Check sheet for the modelled part. Datum: model origin and axes. Units: mm. Round coordinates to 2 decimals unless told otherwise and drop trailing zeros. Write each loop counter-clockwise with the first axis right and the second up, starting at its lowest first coordinate (ties: lowest second). Pieces come first, ordered by that corner, then holes.
Item 1: Material ranges on line 1 along X through (y, z) = (52.5, 1.5); line 2 along Y through (x, z) = (-206, 2.25); line 3 along Y through (x, z) = (-303, 4.5), recorded low to high.
Item 2: Section check B-B, the plane x = -58.5. Record the cut outline in (y, z).
Item 3: Section check A-A, the plane y = 93.5. Record the cut outline in (x, z).
Item 4: Section check D-D, the plane x = 269. Record the cut outline in (y, z), plus the area to 3 significant figures.
Item 5: Depth check by flat-ended pin: pin 1 (1 mm diameter, centred on x = 224.5, z = 1, fed in from +Y); pin 2 (3.5 mm diameter, centred on x = 45, z = 0.5, fed in from +Y); pin 3 (3 mm diameter, centred on y = 11, z = -1.5, fed in from -X); pin 4 (4 mm diameter, centred on x = 169.5, y = 18.5, fed in from -Z). Enter the tip coordinate at first touch or a pass-through.
Item 6: Release check for a two-part mould opening along Y. For faces 1 (the flat face through (234.723, 149.645, 0.067)), 2 (the flat face through (80, 89, 4.762)), 3 (the cylindrical face through (-214.43, 9.3, -0.07)) record: pulls with the +Y half, pulls with the -Y half, needs draft (parallel to the pull), parting line crosses it, or undercut.
Item 7: Section check C-C, the plane z = 0. State how many separate pieces and enclosed holes the cut face has, plus the area to 3 significant figures.
from build123d import *

# Parameters (mm, degrees)
SKETCH2_R           = 7.239
BOSS_EXTRUDE1_DEPTH = 4.7625
FILLET1_R           = 25.4
FILLET2_R           = 101.6
SKETCH3_W           = 25.4
SKETCH3_H           = 27.686
CUT_EXTRUDE1_DEPTH  = 10.525
SKETCH5_W           = 88.9
SKETCH5_H           = 114.3
CUT_EXTRUDE2_DEPTH  = 10.525
CUT_EXTRUDE3_DEPTH  = 10.525


with BuildPart() as part:
    # Sketch2 → Boss-Extrude1 (new body, symmetric)
    with BuildSketch(Plane.XY):
        Polygon((-340, 26.400000032), (-340, 121.400000032), (-75, 165), (135, 176.400000032), (340, 121.400000032), (340, 26.400000032), (340, 0), (-340, 0), align=None)
        with Locations((-208.682, 13.700000032)):
            Circle(SKETCH2_R, mode=Mode.SUBTRACT)
        with Locations((-77.364, 13.700000032)):
            Circle(SKETCH2_R, mode=Mode.SUBTRACT)
        with Locations((53.954, 13.700000032)):
            Circle(SKETCH2_R, mode=Mode.SUBTRACT)
        with Locations((185.126699107, 12.7)):
            Circle(SKETCH2_R, mode=Mode.SUBTRACT)
        with Locations((306.284699107, 10.414)):
            Circle(SKETCH2_R, mode=Mode.SUBTRACT)
        with Locations((168.225103232, 12.7)):
            Circle(SKETCH2_R, mode=Mode.SUBTRACT)
    extrude(amount=BOSS_EXTRUDE1_DEPTH, both=True)

    # Fillet1
    fillet1_edges = [part.edges().sort_by_distance(p)[0] for p in [
        (-340, 121.400000032, 0),
        (340, 121.400000032, 0),
    ]]
    fillet(fillet1_edges, radius=FILLET1_R)

    # Fillet2
    fillet2_edges = [part.edges().sort_by_distance(p)[0] for p in [
        (-75, 165, 0),
        (135, 176.400000032, 0),
    ]]
    fillet(fillet2_edges, radius=FILLET2_R)

    # Sketch3 → Cut-Extrude1 (cut, through all)
    with BuildSketch(Plane.XY.offset(4.7625)):
        with Locations((-327.3, 13.843)):
            Rectangle(SKETCH3_W, SKETCH3_H)
    extrude(amount=-CUT_EXTRUDE1_DEPTH, mode=Mode.SUBTRACT)

    # Sketch5 → Cut-Extrude2 (cut, through all)
    with BuildSketch(Plane.XY.offset(4.7625)):
        with Locations((-36.66848567, 86.296499999)):
            Rectangle(SKETCH5_W, SKETCH5_H)
    extrude(amount=-CUT_EXTRUDE2_DEPTH, mode=Mode.SUBTRACT)

    # Sketch8 → Cut-Extrude3 (cut, through all)
    with BuildSketch(Plane.XY.offset(4.7625)):
        with BuildLine():
            Line((161, 37.4), (162, 37.4))
            ThreePointArc((162, 37.4), (164.1, 35.3), (162, 33.2))
            Line((162, 33.2), (161, 33.2))
            ThreePointArc((161, 33.2), (158.9, 35.3), (161, 37.4))
        make_face()
        with BuildLine():
            Line((47, 33.2), (44, 33.2))
            ThreePointArc((44, 33.2), (41.9, 35.3), (44, 37.4))
            Line((44, 37.4), (47, 37.4))
            ThreePointArc((47, 37.4), (49.1, 35.3), (47, 33.2))
        make_face()
    extrude(amount=-CUT_EXTRUDE3_DEPTH, mode=Mode.SUBTRACT)


solid = part.part
Values found:
1. line 1: x = -340 to -81.12, 7.78 to 340
1. line 2: y = 0 to 6.98, 20.42 to 143.45
1. line 3: y = 0 to 127.49
2. outline: (0, -4.76) - (29.15, -4.76) - (29.15, 4.76) - (0, 4.76) - close; (143.45, -4.76) - (165.9, -4.76) - (165.9, 4.76) - (143.45, 4.76) - close
3. outline: (-340, -4.76) - (-81.12, -4.76) - (-81.12, 4.76) - (-340, 4.76) - close; (7.78, -4.76) - (340, -4.76) - (340, 4.76) - (7.78, 4.76) - close
4. outline: (0, -4.76) - (140.45, -4.76) - (140.45, 4.76) - (0, 4.76) - close
4. area: 1,340 mm2
5. pin 1: stops at y = 152.52
5. pin 2: stops at y = 171.61
5. pin 3: stops at x = -314.6
5. pin 4: stops at z = -4.76
6. face 1: pulls with the +Y half
6. face 2: needs draft
6. face 3: undercut
7. separate pieces: 1
7. enclosed holes: 9
7. area: 92,200 mm2
